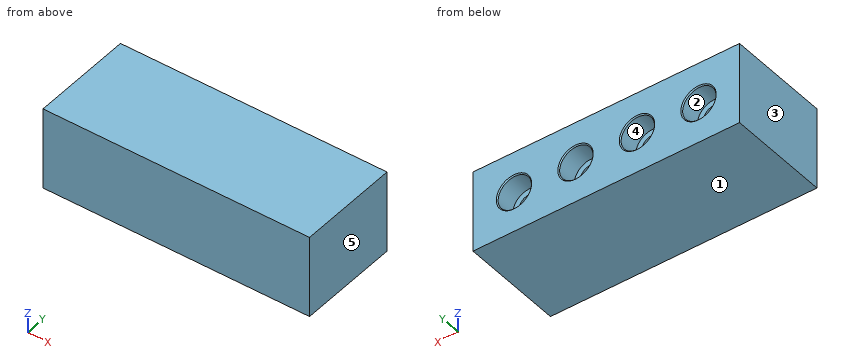
from build123d import *

# Parameters (mm, degrees)
SKETCH1_W           = 165.1
SKETCH1_H           = 63.5
BOSS_EXTRUDE1_DEPTH = 25.4
LPATTERN1_COUNT     = 4
LPATTERN1_PITCH     = 38.1


with BuildPart() as part:
    # Sketch1 → Boss-Extrude1 (new body, symmetric)
    with BuildSketch(Plane.XY):
        Rectangle(SKETCH1_W, SKETCH1_H)
    extrude(amount=BOSS_EXTRUDE1_DEPTH, both=True)

    # Sketch4 → CBORE for 1/2 Socket Head Cap Screw2 (revolve, cut)
    with BuildSketch(Plane(origin=(-57.15, 31.75, 0), x_dir=(0, 0, 1), z_dir=(1, 0, 0))):
        Polygon((0, 0), (0, 54.853549943), (6.74624, 50.8), (6.74624, 12.7), (10.31875, 12.7), (10.31875, 0.635), (10.95375, 0), align=None)
    cbore_for_1_2_socket_head_cap_screw2 = revolve(axis=Axis((-57.15, 38.1, 0), (0, -1, 0)), mode=Mode.SUBTRACT)

    # LPattern1: CBORE for 1/2 Socket Head Cap Screw2 ×4
    with Locations(*[(i * LPATTERN1_PITCH, 0, 0) for i in range(1, LPATTERN1_COUNT)]):
        add(cbore_for_1_2_socket_head_cap_screw2, mode=Mode.SUBTRACT)


solid = part.part
Verification items for the finished model (mm, model axes). Face numbers are marked on the shaded views. A direction names the side the tool comes from. Coordinates: 2 decimals unless noted, no trailing zeros. Loops run counter-clockwise (first coordinate to the right, second up) from the corner with the lowest first, then second, coordinate; pieces in that order, holes last. Notation, with made-up numbers: (-29, -18.5) -> (4, -18.5) arc R19 ccw to (4, 0.5) -> close; hole circle Ø10 at (20, 25.25). An arc over 180 degrees is marked (long way). Answer as a JSON object with one key per item and string values. Group by question number.
Item 1: Sectioned sample at A-A on y = 7. Record the boundary of the cut face in (x, z).
Item 2: Scan lines: probe 1 along X at (y, z) = (21.75, 0); probe 2 along X at (y, z) = (7, 0); probe 3 along Z at (x, y) = (-57.15, 9.5). Record each from-to range of solid material in increasing order.
Item 3: Depth check by flat-ended pin: pin 1 (6 mm diameter, centred on x = 59, z = 5, fed in from +Y); pin 2 (12 mm diameter, centred on x = -57.15, z = 0, fed in from +Y); pin 3 (21.5 mm diameter, centred on x = -19.05, z = 0, fed in from +Y). Enter the tip coordinate at first touch or a pass-through.
Item 4: Tool access check on the marked faces 4 and 5. Record the directions out of +Z, -Z, +X, -X, +Y, -Y that give a thin tool (end or side, any length) a straight path to the whole face; none if there is none.
Item 5: Mould release check, pull along X, two halves, no side actions. Record for the marked faces 1, 2 and 3: +X half, -X half, draft (parallel to the pull), parting line (faces both ways), or undercut.
Evaluation:
{
 "1": {"outline": "(-82.55, -25.4) -> (82.55, -25.4) -> (82.55, 25.4) -> (-82.55, 25.4) -> close; hole circle Ø13.49 at (-57.15, 0); hole circle Ø13.49 at (-19.05, 0); hole circle Ø13.49 at (19.05, 0); hole circle Ø13.49 at (57.15, 0)"},
 "2": {"probe 1": "x = -82.55 to -67.47, -46.83 to -29.37, -8.73 to 8.73, 29.37 to 46.83, 67.47 to 82.55", "probe 2": "x = -82.55 to -63.9, -50.4 to -25.8, -12.3 to 12.3, 25.8 to 50.4, 63.9 to 82.55", "probe 3": "z = -25.4 to -6.75, 6.75 to 25.4"},
 "3": {"pin 1": "stops at y = 19.05", "pin 2": "stops at y = -19.5", "pin 3": "stops at y = 31.55"},
 "4": {"face 4": "+Y", "face 5": "+Z, -Z, +X, +Y, -Y"},
 "5": {"face 1": "draft", "face 2": "undercut", "face 3": "-X half"}
}
